For this review, take the finished solid that the model builds, in its own axes (mm). Give positions to 0.01 mm unless a question says otherwise; leave off trailing zeros. Loops run counter-clockwise (first coordinate to the right, second up) from the corner with the lowest first, then second, coordinate; pieces in that order, holes last.
```python
from build123d import *

# Parameters (mm, degrees)
F0_W     = 270
F0_H     = 20
F0_R     = 5
F1_DEPTH = 3


with BuildPart() as f1:
    # F0 (on Right) → F1 (new body)
    with BuildSketch(Plane.YZ):
        with Locations((135, 10)):
            Rectangle(F0_W, F0_H)
        with BuildLine():
            ThreePointArc((10, 5), (5, 10), (10, 15))
            Line((10, 15), (56.39484, 15))
            ThreePointArc((56.39484, 15), (59.930374, 13.535534), (61.39484, 10))
            ThreePointArc((61.39484, 10), (59.930374, 6.464466), (56.39484, 5))
            Line((56.39484, 5), (10, 5))
        make_face(mode=Mode.SUBTRACT)
        with BuildLine():
            ThreePointArc((145.45455, 5), (140.45455, 10), (145.45455, 15))
            Line((145.45455, 15), (215.45455, 15))
            ThreePointArc((215.45455, 15), (218.990084, 13.535534), (220.45455, 10))
            ThreePointArc((220.45455, 10), (218.990084, 6.464466), (215.45455, 5))
            Line((215.45455, 5), (145.45455, 5))
        make_face(mode=Mode.SUBTRACT)
        with Locations((260, 10)):
            Circle(F0_R, mode=Mode.SUBTRACT)
    extrude(amount=F1_DEPTH)


solid = f1.part
```
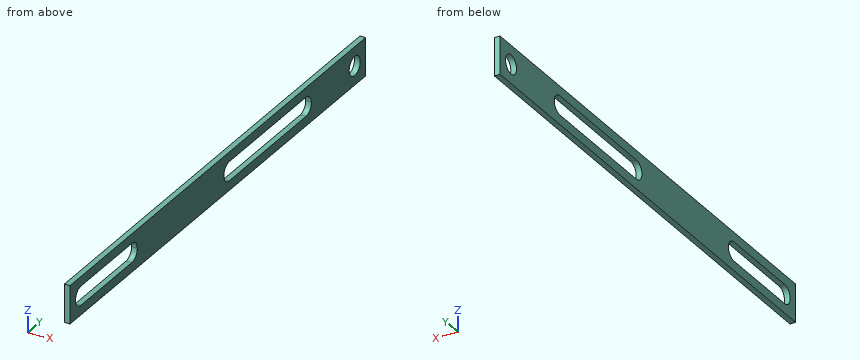
Q1. For probe 1 along Z at (x, y) = (0.7, 260); probe 2 along Y at (x, z) = (1.45, 9); probe 3 along Y at (x, z) = (2.5, 11.25), list the stretches that pass through material, from the lowest coordinate up.
Answers:
probe 1: z = 0 to 5, 15 to 20
probe 2: y = 0 to 5.1, 61.29 to 140.56, 220.35 to 255.1, 264.9 to 270
probe 3: y = 0 to 5.16, 61.24 to 140.61, 220.3 to 255.16, 264.84 to 270
Q2. Consider section A-A on x = 2.15. Give the boundary of the cut face in (y, z), plus the area to 3 significant figures.
Answers:
outline: (0, 0) - (270, 0) - (270, 20) - (0, 20) - close; hole (10, 5) - (56.39, 5) arc R5 ccw to (56.39, 15) - (10, 15) arc R5 ccw to start; hole (145.45, 5) - (215.45, 5) arc R5 ccw to (215.45, 15) - (145.45, 15) arc R5 ccw to start; hole circle Ø10 at (260, 10)
area: 4,000 mm2
Q3. Consider section B-B on y = 191. Give the boundary of the cut face in (x, z).
Answers:
outline: (0, 0) - (3, 0) - (3, 5) - (0, 5) - close; (0, 15) - (3, 15) - (3, 20) - (0, 20) - close
Q4. For pin 1 Ø8 at (y, z) = (260, 10) entering from +X; pin 2 Ø3 at (y, z) = (203, 3) entering from -X, all flat-tipped, find the tip position at first contact; note any pin that passes through.
Answers:
pin 1: passes through
pin 2: stops at x = 0
